Could you check a few things on this model? Use its own coordinates, in mm. A direction names the side the tool comes from. Round coordinates to 2 decimals unless told otherwise and drop trailing zeros. Loops run counter-clockwise (first coordinate to the right, second up) from the corner with the lowest first, then second, coordinate; pieces in that order, holes last. Notation, with made-up numbers: (13, 63.25) -> (43, 63.25) arc R11 ccw to (43, 79.25) -> close; hole circle Ø2 at (-15, 46.5). An arc over 180 degrees is marked (long way). One line per item, written item: value.
```python
from build123d import *

# Parameters (mm, degrees)
SKETCH_3_W          = 14.74967026
SKETCH_3_H          = 24.956193141
CUT_EXTRUDE_2_DEPTH = 18
EXTRUDE_2_DEPTH     = 1.5
FILLET_1_R          = 2


with BuildPart() as part:
    # 草图1 → 旋转1 (revolve)
    with BuildSketch(Plane.XY, mode=Mode.PRIVATE) as revolve_1_sk:
        Polygon((-11.6, 6), (-11.6, 14), (-23, 14), (-23, 12), (-20, 13), (-20, 11), (-17, 11), (-17, 7.4), (-13, 7.4), (-13, 6), align=None)
    revolve(revolve_1_sk.sketch.rotate(Axis((-19.18351236, 2.5, 0), (1, 0, 0)), 180), axis=Axis((-19.18351236, 2.5, 0), (1, 0, 0)))

    # 草图3 → 切除-拉伸2 (cut)
    with BuildSketch(Plane.XY):
        with Locations((-16.988825522, 2.302922831)):
            Rectangle(SKETCH_3_W, SKETCH_3_H)
    extrude(amount=-CUT_EXTRUDE_2_DEPTH, mode=Mode.SUBTRACT)

    # 草图4 → 凸台-拉伸2 (add)
    with BuildSketch(Plane(origin=(0, 0, 0), x_dir=(-1, 0, 0), z_dir=(0, 0, -1))):
        with BuildLine():
            Line((14.8, 14), (14.8, 19.45))
            Line((14.8, 19.45), (17.1, 19.45))
            Line((17.1, 19.45), (17.1, 18.436140662))
            ThreePointArc((17.1, 18.436140662), (17.3, 15.55), (17.5, 18.436140662))
            Line((17.5, 18.436140662), (17.5, 19.45))
            Line((17.5, 19.45), (19.8, 19.45))
            Line((19.8, 19.45), (19.8, 14))
            Line((19.8, 14), (19.8, 12.669411603))
            Line((19.8, 12.669411603), (14.8, 12.669411603))
            Line((14.8, 12.669411603), (14.8, 14))
        make_face()
        with BuildLine():
            Line((19.8, -9), (19.8, -7.669411603))
            Line((19.8, -7.669411603), (14.8, -7.669411603))
            Line((14.8, -7.669411603), (14.8, -9))
            Line((14.8, -9), (14.8, -14.45))
            Line((14.8, -14.45), (17.1, -14.45))
            Line((17.1, -14.45), (17.1, -13.436140662))
            ThreePointArc((17.1, -13.436140662), (17.3, -10.55), (17.5, -13.436140662))
            Line((17.5, -13.436140662), (17.5, -14.45))
            Line((17.5, -14.45), (19.8, -14.45))
            Line((19.8, -14.45), (19.8, -9))
        make_face()
    extrude(amount=-EXTRUDE_2_DEPTH)

    # 圆角1
    fillet_1_edges = [part.edges().sort_by_distance(p)[0] for p in [
        (-11.6, 2.5, 11.5),
    ]]
    fillet(fillet_1_edges, radius=FILLET_1_R)


solid = part.part
```
Item 1: If we mould it in two halves opening along Y, with no side actions, what happens to faces 1 (the face through (-11.6, 2, 5)), 2 (the face through (-19, 19.45, 1)), 3 (the face through (-15, 2.6, 4.9))? For each: released by +Y, released by -Y, zero draft, split by the parting line, or undercut.
Output:
face 1: zero draft
face 2: released by +Y
face 3: undercut
Item 2: Will these pins go through, and if not, where does the flat tip stop? pin 1 Ø4 at (y, z) = (12, 7.5) entering from +X; pin 2 Ø5.5 at (x, y) = (-18, 18) entering from +Z; pin 3 Ø3 at (x, y) = (-16, 1.5) entering from -Z.
Output:
pin 1: stops at x = -11.69
pin 2: stops at z = 1.5
pin 3: stops at z = 4.21
Item 3: I need wall thicknesses on line 1 (X direction, y = -12, z = 1); line 2 (Y direction, x = -16, z = 1); line 3 (Z direction, x = -14.25, y = 2.5). Which ranges of each line are inside material? Lowest first, please. Write a range as from..to.
Output:
line 1: x = -19.8..-18.75, -15.85..-14.8
line 2: y = -14.45..-12.64, -11.36..-2.3, 7.3..16.36, 17.64..19.45
line 3: z = 4.9..11.5
Item 4: If we section it at A-A on y = -11: List the corners of the cut face in (x, z) for me, plus the area to 3 significant figures.
Output:
outline: (-19.8, 0) -> (-18.35, 0) -> (-18.35, 1.5) -> (-19.8, 1.5) -> close; (-16.25, 0) -> (-14.8, 0) -> (-14.8, 1.5) -> (-16.25, 1.5) -> close
area: 4.35 mm²
Item 5: If we section it at B-B on y = 17: List the corners of the cut face in (x, z) for me, plus the area to 3 significant figures.
Output:
outline: (-19.8, 0) -> (-18.75, 0) -> (-18.75, 1.5) -> (-19.8, 1.5) -> close; (-15.85, 0) -> (-14.8, 0) -> (-14.8, 1.5) -> (-15.85, 1.5) -> close
area: 3.15 mm²
Item 6: For faces 4 (the face through (-22.48, 2.71, 9.67)), 5 (the face through (-18.479, 2.687, 8.498)), 6 (the face through (-17.5, -14, 1)), 7 (the face through (-17.1, 19, 1)), which set-ups out of +Z, -Z, +X, -X, +Y, -Y let a thin tool reach every point of the face, with its end or its side?
Output:
face 4: -Z
face 5: -Z, -X
face 6: +Z, -Z, -Y
face 7: +Z, -Z, +Y
Item 7: If we section it at C-C on x = -20.5: List the corners of the cut face in (y, z) for me, plus the area to 3 significant figures.
Output:
outline: (-9, 0) -> (-7.83, 0) arc R10.33 cw to (12.83, 0) -> (14, 0) arc R11.5 ccw to start
area: 40.0 mm²
